Can you work these out from the model? Positions are in its coordinate system, mm. Face numbers are marked on the shaded views. A direction names the side the tool comes from. Round coordinates to 2 decimals unless told otherwise and drop trailing zeros. Order: outer loops, then holes, each group sorted by start corner. A loop starts at its lowest first (then second) coordinate and runs counter-clockwise, first axis right, second up. Notation, with made-up numbers: (-33, -15.75) -> (-7, -15.75) arc R26 cw to (-7, 23.25) -> close; hole circle Ø7 at (75, 2.5). An arc over 180 degrees is marked (long way). One line per item, written item: value.
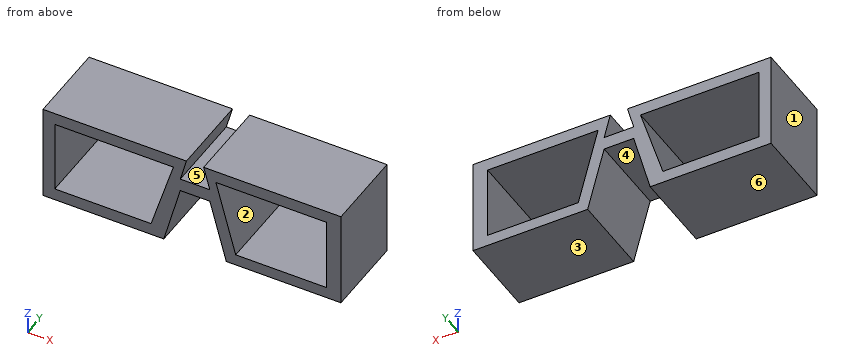
```python
from build123d import *

# Parameters (mm, degrees)
F1_DEPTH = 25


with BuildPart() as f1:
    # F0 (on Front) → F1 (new body)
    with BuildSketch(Plane.XZ):
        Polygon((42.044164, -7.025787), (43.926718, 0), (0, 0), (0, -29.861876), (36.991882, -29.861876), (42.044164, -11.006502), (51.090819, -11.006502), (56.143101, -29.861876), (91.252429, -29.861876), (91.252429, 0), (49.208265, 0), (51.090819, -7.025787), align=None)
        Polygon((3.600854, -26.124269), (3.600854, -3.742162), (39.94265, -3.742162), (33.090983, -26.124269), align=None, mode=Mode.SUBTRACT)
        Polygon((52.949521, -3.742162), (86.779835, -3.742162), (86.779835, -26.366743), (59.011759, -26.366743), align=None, mode=Mode.SUBTRACT)
    extrude(amount=F1_DEPTH)


solid = f1.part
```
Q1. Please list where these lines run through material, in increasing order: line 1 along Z through (x, y) = (25, -10.5); line 2 along Z through (x, y) = (72, -7.75); line 3 along X through (y, z) = (-12.25, -21).
Answers below:
line 1: -29.86 to -26.12, -3.74 to 0
line 2: -29.86 to -26.37, -3.74 to 0
line 3: 0 to 3.6, 34.66 to 39.37, 53.77 to 57.57, 86.78 to 91.25
Q2. I want a section at B-B on x = 54.5. List the corners of the cut face in (y, z) for me.
Answers below:
outline: (-25, -23.73) -> (0, -23.73) -> (0, -9.53) -> (-25, -9.53) -> close; (-25, -3.74) -> (0, -3.74) -> (0, 0) -> (-25, 0) -> close
Q3. I want a section at C-C on z = -20.75. List the corners of the cut face in (x, y) for me.
Answers below:
outline: (0, -25) -> (3.6, -25) -> (3.6, 0) -> (0, 0) -> close; (34.74, -25) -> (39.43, -25) -> (39.43, 0) -> (34.74, 0) -> close; (53.7, -25) -> (57.51, -25) -> (57.51, 0) -> (53.7, 0) -> close; (86.78, -25) -> (91.25, -25) -> (91.25, 0) -> (86.78, 0) -> close
Q4. On a 3-axis mill with a long thin cutter (end or side, diameter ignored), from which of +Z, -Z, +X, -X, +Y, -Y can I reach the whole of each face in a straight line? I mean the marked faces 4, 5 and 6. Say none if no direction works.
Answers below:
face 4: -Z, +Y, -Y
face 5: +Y, -Y
face 6: -Z, +X, -X, +Y, -Y
Q5. We'd pull the mould along X, two halves only. Please class the marked faces 1, 2 and 3: released by +X, released by -X, zero draft, split by the parting line, or undercut.
Answers below:
face 1: released by -X
face 2: undercut
face 3: zero draft
Q6. Will these pins go through, and if not, where does the flat tip stop? pin 1 Ø4.5 at (x, y) = (44.5, -10.5) entering from -Z; pin 2 Ø4.5 at (x, y) = (46.5, -6.5) entering from +Z.
Answers below:
pin 1: z = -11.01
pin 2: z = -7.03
Q7. I want a section at D-D on x = 72. List the corners of the cut face in (y, z) for me.
Answers below:
outline: (-25, -29.86) -> (0, -29.86) -> (0, -26.37) -> (-25, -26.37) -> close; (-25, -3.74) -> (0, -3.74) -> (0, 0) -> (-25, 0) -> close
Q8. I want a section at A-A on y = -17.25. List the corners of the cut face in (x, z) for me, plus the area to 3 significant figures.
Answers below:
outline: (0, -29.86) -> (36.99, -29.86) -> (42.04, -11.01) -> (51.09, -11.01) -> (56.14, -29.86) -> (91.25, -29.86) -> (91.25, 0) -> (49.21, 0) -> (51.09, -7.03) -> (42.04, -7.03) -> (43.93, 0) -> (0, 0) -> close; hole (3.6, -26.12) -> (33.09, -26.12) -> (39.94, -3.74) -> (3.6, -3.74) -> close; hole (52.95, -3.74) -> (59.01, -26.37) -> (86.78, -26.37) -> (86.78, -3.74) -> close
area: 975 mm^2
